```python
from build123d import *

# Parameters (mm, degrees)
EXTRUDE_1_DEPTH = 8
CHAMFER_1_SIZE  = 0.4
CHAMFER_2_SIZE  = 0.4


with BuildPart() as part:
    # 草图1 → 凸台-拉伸1 (new body)
    with BuildSketch(Plane(origin=(0, 0, 0), x_dir=(1, 0, 0), z_dir=(0, 1, 0))):
        with BuildLine():
            Line((-12, 6), (12, 6))
            ThreePointArc((12, 6), (18, 0), (12, -6))
            Line((12, -6), (-12, -6))
            ThreePointArc((-12, -6), (-18, 0), (-12, 6))
        make_face()
    extrude(amount=EXTRUDE_1_DEPTH)

    # 倒角1
    chamfer_1_edges = [part.edges().sort_by_distance(p)[0] for p in [
        (18, 8, 0),
        (0, 8, -6),
        (-18, 8, 0),
        (0, 8, 6),
    ]]
    chamfer(chamfer_1_edges, length=CHAMFER_1_SIZE)

    # 倒角2
    chamfer_2_edges = [part.edges().sort_by_distance(p)[0] for p in [
        (0, 0, -6),
        (18, 0, 0),
        (0, 0, 6),
        (-18, 0, 0),
    ]]
    chamfer(chamfer_2_edges, length=CHAMFER_2_SIZE)


solid = part.part
```
For this review, take the finished solid that the model builds, in its own axes (mm). Round coordinates to 2 decimals unless told otherwise and drop trailing zeros. Order: outer loops, then holes, each group sorted by start corner. A loop starts at its lowest first (then second) coordinate and runs counter-clockwise, first axis right, second up.
Q1. Wall thickness on line 1 (X direction, y = 3.25, z = 1.5); line 2 (Z direction, x = 12.5, y = 7.75); line 3 (X direction, y = 7.25, z = -0.5): over which ranges is each line inside the solid? List them lowest first.
Findings below:
line 1: x = -17.81 to 17.81
line 2: z = -5.83 to 5.83
line 3: x = -17.98 to 17.98
Q2. Insertion check: P1, Ø3, axis at y = 4, z = 3, coming from the -X side. The pin has a flat end and moves straight along its axis. Give the tip position at first contact, or say it passes through.
Findings below:
P1: stops at x = -17.81
Q3. We need section A-A, the plane y = 2.25. Give the boundary of the cut face in (x, z).
Findings below:
outline: (-12, -6) - (12, -6) arc R6 ccw to (12, 6) - (-12, 6) arc R6 ccw to start
